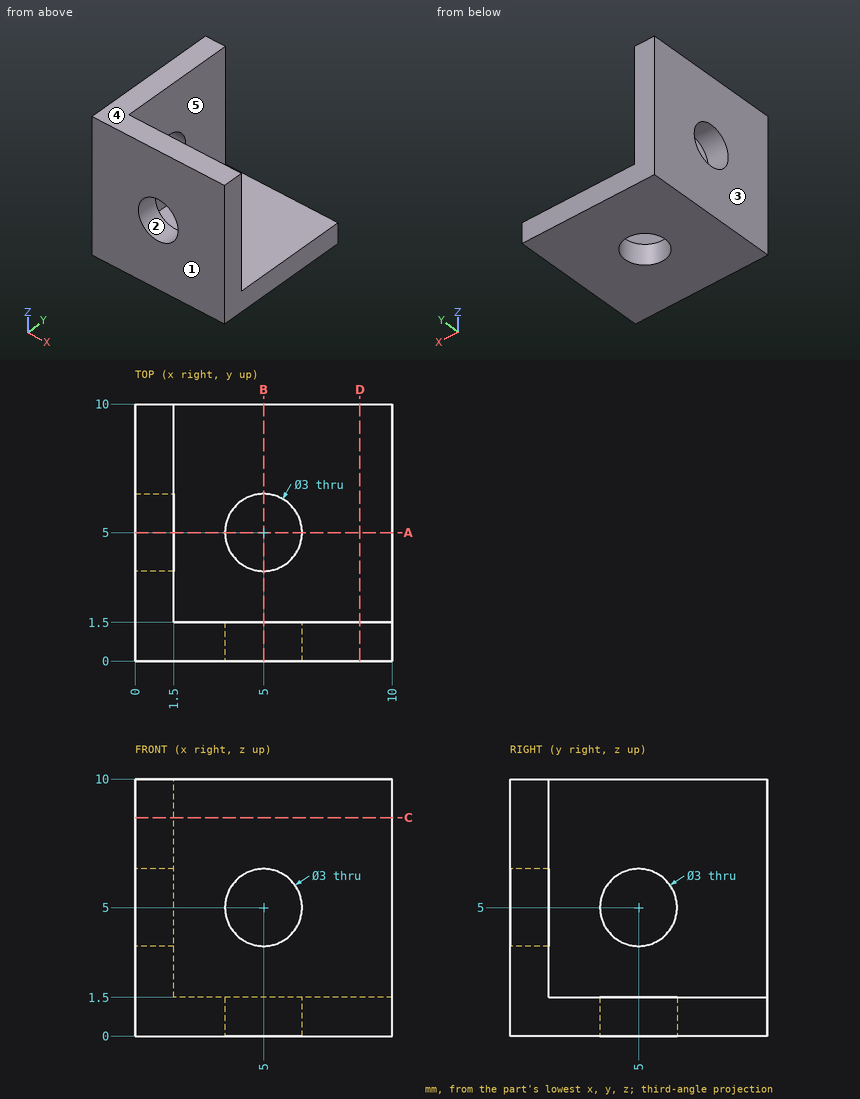
Input: dimensioned drawing with shaded views. Units: mm. Origin: part minimum x, y, z. A direction names the side the tool comes from. Round coordinates to 2 decimals unless told otherwise and drop trailing zeros. Order: outer loops, then holes, each group sorted by start corner. A loop starts at its lowest first (then second) coordinate and runs counter-clockwise, first axis right, second up. Notation, with made-up numbers: (-2.75, 50.5) - (45.25, 50.5) arc R29 ccw to (45.25, 83.5) - close; hole circle Ø2 at (-28, -30). An arc over 180 degrees is marked (long way). Answer as a JSON object with one key per item and string values. Group by question number.
(1) Reachability of the marked faces 4 and 5 from +Z, -Z, +X, -X, +Y, -Y: full face, straight path, thin tool, end or side. Return the list, or none.
(2) Pin query (flat end, axial travel): P1, Ø2.5, axis at x = 3.5, y = 4, coming from the +Z side; P2, Ø5, axis at x = 5, z = 5, coming from the +Y side. Return the tip coordinate at first contact, or that it passes through.
(3) Draft query along X for the marked faces 1, 2 and 3. Return one class per face: released by +X, released by -X, zero draft, split by the parting line, or undercut.
(4) Material intervals for probe 1 along Z at (x, y) = (5, 0.65); probe 2 along Y at (x, z) = (8, 9.75), sorted ascending. Write a range as from..to.
(5) Cut plane A-A (y = 5). Return loops of the section in (x, z).
(6) Cut plane C-C (z = 8.5). Return loops of the section in (x, y).
Here are the results:
{
 "1": {"face 4": "+Z, +X, -X, +Y, -Y", "face 5": "+Z, +X, +Y"},
 "2": {"P1": "stops at z = 1.5", "P2": "stops at y = 1.5"},
 "3": {"face 1": "zero draft", "face 2": "undercut", "face 3": "released by -X"},
 "4": {"probe 1": "z = 0..3.5, 6.5..10", "probe 2": "y = 0..1.5"},
 "5": {"outline": "(0, 0) - (3.5, 0) - (3.5, 1.5) - (1.5, 1.5) - (1.5, 3.5) - (0, 3.5) - close; (0, 6.5) - (1.5, 6.5) - (1.5, 10) - (0, 10) - close; (6.5, 0) - (10, 0) - (10, 1.5) - (6.5, 1.5) - close"},
 "6": {"outline": "(0, 0) - (10, 0) - (10, 1.5) - (1.5, 1.5) - (1.5, 10) - (0, 10) - close"}
}
